The listing builds one solid part. Answer for the finished solid, in the listing's coordinates (mm). A direction names the side the tool comes from. Coordinates: 2 decimals unless noted, no trailing zeros. Loops run counter-clockwise (first coordinate to the right, second up) from the corner with the lowest first, then second, coordinate; pieces in that order, holes last. Notation, with made-up numbers: M 12.25,-8 L 41.25,-8 A36 ccw 41.25,31 Z; hole C 39,-16 d4. An arc over 180 degrees is marked long. Answer as a JSON object with one key per item and string values. Group by question number.
1. A cutting plane is placed at C-C on y = 5.75. Give the vertices of the cut face in (x, z), and give its area (3 significant figures).
2. A cutting plane is placed at D-D on y = 9.75. Give the vertices of the cut face in (x, z), and give its area (3 significant figures).
3. A cutting plane is placed at B-B on z = 3.5. Give the vertices of the cut face in (x, y), and give its area (3 significant figures).
4. A cutting plane is placed at A-A on x = -3.5. Give the vertices of the cut face in (y, z), and give its area (3 significant figures).
5. Straight lines are drawn through the part: L1, parallel to X at y = 10, z = 3.5; L2, parallel to X at y = 14.5, z = 3.5; L3, parallel to X at y = 8.5, z = 3. For each, find the intervals that lie inside material, in ascending order.
6. Given pin 1 (1.6 mm diameter, centred on x = 3.5, z = 3.5, fed in from +Y); pin 2 (4 mm diameter, centred on y = 0, z = 6, fed in from +X); pin 3 (3 mm diameter, centred on x = -3.5, z = 3.5, fed in from +Y); pin 4 (1.8 mm diameter, centred on x = 9.5, z = 3.5, fed in from -Y), each flat-ended and moving along its own axis, determine where each tip first touches the part or whether it passes through.
7. Determine the mould class of faces 1 (the face through (-5, 6.5, 2)), 2 (the face through (2, 4, 0)), 3 (the face through (0, -4, 4)) for opening direction Z: released by +Z, released by -Z, zero draft, split by the parting line, or undercut.
8. For faces 4 (the face through (2.3, 9.84, 4.12)), 5 (the face through (-2, 9.5, 1)), 6 (the face through (10, 15.75, 3)), 7 (the face through (9, 13.75, 3)), 8 (the face through (-7, 3, 3)), determine the directions among +Z, -Z, +X, -X, +Y, -Y from which every point of the face is accessible in a straight line to the end or side of a thin tool.
from build123d import *

# Parameters (mm, degrees)
SALIENTE_EXTRUIR1_DEPTH = 7
CROQUIS4_R              = 1.35
CORTAR_EXTRUIR1_DEPTH   = 13.5
CROQUIS5_R              = 1.6
CORTAR_EXTRUIR2_DEPTH   = 13.9
CROQUIS6_R              = 2.75
CORTAR_EXTRUIR3_DEPTH   = 3
CROQUIS7_W              = 11
CROQUIS7_H              = 7
CROQUIS7_R              = 1.6
SALIENTE_EXTRUIR2_DEPTH = 4


with BuildPart() as part:
    # Croquis1 → Saliente-Extruir1 (new body)
    with BuildSketch(Plane.XY):
        Polygon((0, 0), (4, 0), (4, -4), (7, -4), (7, 0), (7, 13.75), (10.5, 13.75), (10.5, 15.75), (9.5, 15.75), (9.5, 16.5), (7, 16.5), (0, 16.5), (0, 9.5), (-7, 9.5), (-7, 0), align=None)
    extrude(amount=SALIENTE_EXTRUIR1_DEPTH)

    # Croquis4 → Cortar-Extruir1 (cut)
    with BuildSketch(Plane(origin=(0, 16.5, 0), x_dir=(1, 0, 0), z_dir=(0, 1, 0))):
        with Locations(Location((3.5, -3.5, 0), (0, 0, 270))):
            Circle(CROQUIS4_R)
    extrude(amount=-CORTAR_EXTRUIR1_DEPTH, mode=Mode.SUBTRACT)

    # Croquis5 → Cortar-Extruir2 (cut)
    with BuildSketch(Plane(origin=(0, 9.5, 0), x_dir=(1, 0, 0), z_dir=(0, 1, 0))):
        with Locations(Location((-3.5, -3.5, 0), (0, 0, 180))):
            Circle(CROQUIS5_R)
    extrude(amount=-CORTAR_EXTRUIR2_DEPTH, mode=Mode.SUBTRACT)

    # Croquis6 → Cortar-Extruir3 (cut)
    with BuildSketch(Plane(origin=(0, 9.5, 0), x_dir=(1, 0, 0), z_dir=(0, 1, 0))):
        with Locations(Location((-3.5, -3.5, 0), (0, 0, 180))):
            Circle(CROQUIS6_R)
    extrude(amount=-CORTAR_EXTRUIR3_DEPTH, mode=Mode.SUBTRACT)

    # Croquis7 → Saliente-Extruir2 (add)
    with BuildSketch(Plane.XZ):
        with Locations((-1.5, 3.5)):
            Rectangle(CROQUIS7_W, CROQUIS7_H)
        with Locations(Location((-3.5, 3.5, 0), (0, 0, 180))):
            Circle(CROQUIS7_R, mode=Mode.SUBTRACT)
    extrude(amount=SALIENTE_EXTRUIR2_DEPTH)


solid = part.part
From the geometry:
{
 "1": {"outline": "M -7,0 L 7,0 L 7,7 L -7,7 Z; hole C -3.5,3.5 d3.2; hole C 3.5,3.5 d2.7", "area": "84.2 mm²"},
 "2": {"outline": "M 0,0 L 7,0 L 7,7 L 0,7 Z; hole C 3.5,3.5 d2.7", "area": "43.3 mm²"},
 "3": {"outline": "M -7,-4 L -5.1,-4 L -5.1,6.5 L -6.25,6.5 L -6.25,9.5 L -7,9.5 Z; M -1.9,-4 L 7,-4 L 7,13.75 L 10.5,13.75 L 10.5,15.75 L 9.5,15.75 L 9.5,16.5 L 4.85,16.5 L 4.85,3 L 2.15,3 L 2.15,16.5 L 0,16.5 L 0,9.5 L -0.75,9.5 L -0.75,6.5 L -1.9,6.5 Z", "area": "160 mm²"},
 "4": {"outline": "M -4,0 L 9.5,0 L 9.5,0.75 L 6.5,0.75 L 6.5,1.9 L -4,1.9 Z; M -4,5.1 L 6.5,5.1 L 6.5,6.25 L 9.5,6.25 L 9.5,7 L -4,7 Z", "area": "44.4 mm²"},
 "5": {"L1": "x = 0 to 2.15, 4.85 to 7", "L2": "x = 0 to 2.15, 4.85 to 10.5", "L3": "x = -7 to -6.2, -0.8 to 2.25, 4.75 to 7"},
 "6": {"pin 1": "stops at y = 3", "pin 2": "stops at x = 7", "pin 3": "passes through", "pin 4": "stops at y = 13.75"},
 "7": {"face 1": "undercut", "face 2": "released by -Z", "face 3": "zero draft"},
 "8": {"face 4": "+Y", "face 5": "+Z, -Z, -X, +Y", "face 6": "+Z, -Z, +X, +Y", "face 7": "+Z, -Z, +X, -Y", "face 8": "+Z, -Z, -X, +Y, -Y"}
}
